Work out the finished part from the listing and answer in its coordinate system (mm). A direction names the side the tool comes from. Coordinates: 2 decimals unless noted, no trailing zeros. Write each loop counter-clockwise with the first axis right and the second up, starting at its lowest first coordinate (ties: lowest second). Pieces come first, ordered by that corner, then holes. Notation, with made-up numbers: M -16,18.25 L 16,18.25 A14 cw 16,27.25 Z; hole C -12.75,40 d6. An arc over 180 degrees is marked long. Answer as CSV lines item,"result". Start each with the question number.
(1) A cutting plane is placed at A-A on y = 81. Give the vertices of the cut face in (x, z), then the cut area to 3 significant figures.
(2) A cutting plane is placed at C-C on x = 26.5. Give the vertices of the cut face in (y, z), then the cut area to 3 significant figures.
(3) The mould has two halves that part along Y. Classify faces 5 (the flat face through (187.813, 50.178, 22.447)), 6 (the flat face through (3, 101.6, 16)), 7 (the flat face through (3, 50, 0)), 8 (the flat face through (3, 0, 16)): released by +Y, released by -Y, zero draft, split by the parting line, or undercut.
(4) For faces 1 (the flat face through (2, 50, 6.35)), 2 (the flat face through (3, 114, 31.75)), 3 (the flat face through (-3, -13, 31.75)), 4 (the flat face through (3, -1, 38.1)), determine the directions among +Z, -Z, +X, -X, +Y, -Y from which every point of the face is accessible in a straight line to the end or side of a thin tool.
(5) A cutting plane is placed at B-B on z = 15.5. Give the vertices of the cut face in (x, y).
(6) Find the intervals of material crossed by L1, parallel to Y at x = -182, z = 31; L2, parallel to Y at x = -137.5, z = 34; L3, parallel to Z at x = -149.5, y = -17, in increasing order. Write a range as [from, to].
(7) A cutting plane is placed at D-D on y = 112. Give the vertices of the cut face in (x, z).
(8) Flat-ended cylindrical pins translate along their axes: P1, Ø5, axis at y = 48.5, z = 5.5, coming from the -X side; P2, Ø1.5, axis at x = -144, y = 17, coming from the +Z side; P3, Ø10, axis at y = 104.5, z = 19, coming from the -X side. Find the tip coordinate at first contact, or state that the pin passes through.
from build123d import *

# Parameters (mm, degrees)
F0_W      = 101.6
F0_H      = 38.1
F1_DEPTH  = 203.2
F3_T      = -6.35
F2_W      = 406.4
F2_H      = 6.35
F4_DEPTH  = 25.4
F5_W      = 406.4
F5_H      = 6.35
F6_DEPTH  = 25.4
F8_DEPTH  = 88.9
F10_DEPTH = 141.224


# Not quite as in the source:
# - a pattern or mirror of a feature is missing from the dataset's text; its kind, count and spacing are read off the source's solid


with BuildPart() as f1:
    # F0 (on Right) → F1 (new body, symmetric)
    with BuildSketch(Plane.YZ):
        with Locations((50.8, 19.05)):
            Rectangle(F0_W, F0_H)
    extrude(amount=F1_DEPTH, both=True)

    # F3
    f3_openings = [f1.faces().sort_by_distance(p)[0] for p in [
        (0, 50.8, 38.1),
    ]]
    offset(amount=F3_T, openings=f3_openings)

    # F2 (on face) → F4 (join)
    with BuildSketch(Plane.XZ):
        with Locations((0, 34.925)):
            Rectangle(F2_W, F2_H)
    extrude(amount=F4_DEPTH)

    # F5 (on face) → F6 (join)
    with BuildSketch(Plane(origin=(0, 101.6, 0), x_dir=(-1, 0, 0), z_dir=(0, 1, 0))):
        with Locations((0, 34.925)):
            Rectangle(F5_W, F5_H)
    extrude(amount=F6_DEPTH)

    # F7 (on face) → F8 (join, through all)
    with BuildSketch(Plane(origin=(0, 6.35, 0), x_dir=(-1, 0, 0), z_dir=(0, 1, 0))):
        Polygon((196.85, 6.35), (196.85, 38.1), (178.5191289532, 6.35), align=None)
    f8 = extrude(amount=F8_DEPTH)

    # F8_copies: F8 across plane
    add(f8.mirror(Plane(origin=(0, 0, 0), x_dir=(0, 0, 1), z_dir=(1, 0, 0))))

    # F9 (on Front) → F10 (cut)
    with BuildSketch(Plane.XZ):
        Polygon((-184.8691289532, 0), (-203.2, 31.75), (-203.2, 0), align=None)
    f10 = extrude(amount=-F10_DEPTH, mode=Mode.SUBTRACT)

    # F10_copies: F10 across plane
    add(f10.mirror(Plane(origin=(0, 0, 0), x_dir=(0, 0, 1), z_dir=(1, 0, 0))), mode=Mode.SUBTRACT)


solid = f1.part
Here are the results:
1,outline,"M -203.2,31.75 L -184.87,0 L 184.87,0 L 203.2,31.75 L 203.2,38.1 L 196.85,38.1 L 178.52,6.35 L -178.52,6.35 L -196.85,38.1 L -203.2,38.1 Z"
1,area,"2,980 mm^2"
2,outline,"M -25.4,31.75 L 0,31.75 L 0,0 L 101.6,0 L 101.6,31.75 L 127,31.75 L 127,38.1 L 95.25,38.1 L 95.25,6.35 L 6.35,6.35 L 6.35,38.1 L -25.4,38.1 Z"
2,area,"1,370 mm^2"
3,face 5,"undercut"
3,face 6,"released by +Y"
3,face 7,"zero draft"
3,face 8,"released by -Y"
4,face 1,"+Z"
4,face 2,"-Z, +X, -X, +Y"
4,face 3,"-Z, +X, -X, -Y"
4,face 4,"+Z, +X, -X, +Y, -Y"
5,outline,"M -193.82,0 L 193.82,0 L 193.82,101.6 L -193.82,101.6 Z; hole M -183.8,6.35 L 183.8,6.35 L 183.8,95.25 L -183.8,95.25 Z"
6,L1,"y = [0, 6.35], [95.25, 101.6]"
6,L2,"y = [-25.4, 6.35], [95.25, 127]"
6,L3,"z = [31.75, 38.1]"
7,outline,"M -203.2,31.75 L 203.2,31.75 L 203.2,38.1 L -203.2,38.1 Z"
8,P1,"stops at x = -189.49"
8,P2,"stops at z = 6.35"
8,P3,"stops at x = -198.19"
